The model under review builds one solid part; all positions refer to its coordinate system, in mm. A direction names the side the tool comes from. Coordinates: 2 decimals unless noted, no trailing zeros. Loops run counter-clockwise (first coordinate to the right, second up) from the corner with the lowest first, then second, coordinate; pieces in that order, holes last. Notation, with made-up numbers: (59.25, -37.5) - (74.25, -37.5) arc R15 ccw to (74.25, -12.5) - close; hole circle Ø8 at (22, -27). An arc over 180 degrees is marked (long way). Use a Markdown table: item, result. Add a question column.
1) To check wall thickness, follow L1, parallel to X at y = 2.7, z = -36.5; L2, parallel to X at y = 5.25, z = 0; L3, parallel to Z at x = -25, y = 1.35. State the ranges of each line that lie inside material, in increasing order. Write a range as [from, to].
2) The part is to be moulded in two halves that separate along Z. For faces 4 (the cylindrical face through (25.428, 1.972, 2.556)), 5 (the flat face through (0, 0, -19)), 6 (the flat face through (-18.5, 7.5, -2.6)), say which applies: pulls with the +Z half, pulls with the -Z half, needs draft (parallel to the pull), parting line crosses it, or undercut.
3) Clearance check with flat-ended pins moving along their axes: pin 1 (2.5 mm diameter, centred on y = 8, z = 0, fed in from -X); pin 2 (6.5 mm diameter, centred on x = -25, z = -36.5, fed in from +Y); pin 3 (1.5 mm diameter, centred on y = 8, z = 0.5, fed in from +X). State where each tip first meets the part, or that it passes through.
4) Add section D-D, the plane z = 11. Give the boundary of the cut face in (x, y), and give its area (3 significant figures).
5) Add section A-A, the plane y = 7.75. Give the boundary of the cut face in (x, z), and give its area (3 significant figures).
6) For faces 1 (the flat face through (21.5, 7.5, 2.6)), 2 (the flat face through (21.5, 7.5, -2.6)), 3 (the flat face through (23, 8, 0)), list the 3-axis set-ups (+Z, -Z, +X, -X, +Y, -Y) from which the entire face can be reached by the end or side of a thin tool; tool diameter is ignored.
7) Add section B-B, the plane z = 0. Give the boundary of the cut face in (x, y), and give its area (3 significant figures).
8) Add section C-C, the plane x = 1. Give the boundary of the cut face in (y, z), and give its area (3 significant figures).
```python
from build123d import *

# Parameters (mm, degrees)
SKETCH1_R           = 14
SKETCH1_R_2         = 2.5
BOSS_EXTRUDE1_DEPTH = 4
FILLET1_R           = 3
SKETCH2_R           = 1.5
CUT_EXTRUDE1_DEPTH  = 10
BOSS_EXTRUDE2_START = 5
SKETCH3_R           = 1.5
BOSS_EXTRUDE2_DEPTH = 5
FILLET2_R           = 2
BOSS_EXTRUDE3_DEPTH = 4


with BuildPart() as part:
    # Sketch1 → Boss-Extrude1 (new body)
    with BuildSketch(Plane(origin=(0, 0, 0), x_dir=(1, 0, 0), z_dir=(0, 1, 0))):
        with BuildLine():
            Line((8.126919667, 17.174200905), (19.588621549, 33.908285652))
            ThreePointArc((19.588621549, 33.908285652), (28.390534034, 41.45017969), (24.538801239, 30.517751618))
            Line((24.538801239, 30.517751618), (13.077099357, 13.783666871))
            ThreePointArc((13.077099357, 13.783666871), (16.116177061, 10.06324187), (18.125, 5.699506558))
            ThreePointArc((18.125, 5.699506558), (26, 0), (18.125, -5.699506558))
            ThreePointArc((18.125, -5.699506558), (11.240760103, -15.318136711), (0, -19))
            ThreePointArc((0, -19), (-11.240760103, -15.318136711), (-18.125, -5.699506558))
            ThreePointArc((-18.125, -5.699506558), (-26, 0), (-18.125, 5.699506558))
            ThreePointArc((-18.125, 5.699506558), (-16.116177061, 10.06324187), (-13.077099357, 13.783666871))
            Line((-13.077099357, 13.783666871), (-24.538801239, 30.517751618))
            ThreePointArc((-24.538801239, 30.517751618), (-28.390534034, 41.45017969), (-19.588621549, 33.908285652))
            Line((-19.588621549, 33.908285652), (-8.126919667, 17.174200905))
            ThreePointArc((-8.126919667, 17.174200905), (0, 19), (8.126919667, 17.174200905))
        make_face()
        with Locations(Location((0, 0, 0), (0, 0, 270))):
            Circle(SKETCH1_R, mode=Mode.SUBTRACT)
        with Locations(Location((25, 36.5, 0), (0, 0, 270))):
            Circle(SKETCH1_R_2, mode=Mode.SUBTRACT)
        with Locations(Location((-25, 36.5, 0), (0, 0, 90))):
            Circle(SKETCH1_R_2, mode=Mode.SUBTRACT)
    extrude(amount=BOSS_EXTRUDE1_DEPTH)

    # Fillet1
    fillet1_edges = [part.edges().sort_by_distance(p)[0] for p in [
        (8.126919667, 2, -17.174200905),
        (19.588621549, 2, -33.908285652),
        (24.538801239, 2, -30.517751618),
        (13.077099357, 2, -13.783666871),
        (18.125, 2, 5.699506558),
        (-18.125, 2, 5.699506558),
        (-18.125, 2, -5.699506558),
        (-13.077099357, 2, -13.783666871),
        (-24.538801239, 2, -30.517751618),
        (-19.588621549, 2, -33.908285652),
        (-8.126919667, 2, -17.174200905),
    ]]
    fillet(fillet1_edges, radius=FILLET1_R)

    # Sketch2 → Cut-Extrude1 (cut)
    with BuildSketch(Plane(origin=(0, 4, 0), x_dir=(1, 0, 0), z_dir=(0, 1, 0))):
        with Locations(Location((20, 0, 0), (0, 0, 270))):
            Circle(SKETCH2_R)
        with Locations(Location((-20, 0, 0), (0, 0, 90))):
            Circle(SKETCH2_R)
    extrude(amount=-CUT_EXTRUDE1_DEPTH, mode=Mode.SUBTRACT)

    # Sketch3 → Boss-Extrude2 (add)
    # profile 1 of 2: a face of its own
    with BuildSketch(Plane(origin=(0, 4, 0), x_dir=(1, 0, 0), z_dir=(0, 1, 0)).offset(BOSS_EXTRUDE2_START)):
        Polygon((-20, 3.464101615), (-23, 1.732050808), (-23, -1.732050808), (-20, -3.464101615), (-17, -1.732050808), (-17, 1.732050808), align=None)
        with Locations(Location((-20, 0, 0), (0, 0, 270))):
            Circle(SKETCH3_R, mode=Mode.SUBTRACT)
    # profile 2 of 2: a face of its own
    with BuildSketch(Plane(origin=(0, 4, 0), x_dir=(1, 0, 0), z_dir=(0, 1, 0)).offset(BOSS_EXTRUDE2_START)):
        Polygon((20, 3.464101615), (17, 1.732050808), (17, -1.732050808), (20, -3.464101615), (23, -1.732050808), (23, 1.732050808), align=None)
        with Locations(Location((20, 0, 0), (0, 0, 270))):
            Circle(SKETCH3_R, mode=Mode.SUBTRACT)
    extrude(amount=-BOSS_EXTRUDE2_DEPTH)

    # Fillet2
    fillet2_edges = [part.edges().sort_by_distance(p)[0] for p in [
        (-18.5, 4, -2.598076211),
        (-21.5, 4, -2.598076211),
        (-23, 4, 0),
        (-21.5, 4, 2.598076211),
        (-18.5, 4, 2.598076211),
        (-17, 4, 0),
        (21.5, 4, -2.598076211),
        (18.5, 4, -2.598076211),
        (17, 4, 0),
        (18.5, 4, 2.598076211),
        (21.5, 4, 2.598076211),
        (23, 4, 0),
    ]]
    fillet(fillet2_edges, radius=FILLET2_R)

    # Sketch4 → Boss-Extrude3 (add)
    with BuildSketch(Plane(origin=(0, 4, 0), x_dir=(1, 0, 0), z_dir=(0, 1, 0))):
        with BuildLine():
            ThreePointArc((24.772139191, 3.636851323), (20.864321919, 18.474065491), (28.618293037, 31.7137744))
            ThreePointArc((28.618293037, 31.7137744), (21.354403975, 32.800609697), (20.161290323, 40.047800538))
            ThreePointArc((20.161290323, 40.047800538), (0, 29.83030278), (-20.161290323, 40.047800538))
            ThreePointArc((-20.161290323, 40.047800538), (-21.354403975, 32.800609697), (-28.618293037, 31.7137744))
            ThreePointArc((-28.618293037, 31.7137744), (-20.864321919, 18.474065491), (-24.772139191, 3.636851323))
            ThreePointArc((-24.772139191, 3.636851323), (-19.807252921, 3.994836175), (-15.415783274, 6.338603052))
            ThreePointArc((-15.415783274, 6.338603052), (-9.04861994, 13.254364925), (0, 15.802110673))
            ThreePointArc((0, 15.802110673), (9.04861994, 13.254364925), (15.415783274, 6.338603052))
            ThreePointArc((15.415783274, 6.338603052), (19.807252921, 3.994836175), (24.772139191, 3.636851323))
        make_face()
    extrude(amount=-BOSS_EXTRUDE3_DEPTH)


solid = part.part
```
From the geometry:
| question | item | result |
|---|---|---|
| 1 | L1 | x = [-31, -27.5], [-22.5, -17], [17, 22.5], [27.5, 31] |
| 1 | L2 | x = [-23.15, -21.5], [-18.5, -16.85], [16.85, 18.5], [21.5, 23.15] |
| 1 | L3 | z = [-42.5, -39], [-34, -28.18], [-3.32, 3.32] |
| 2 | face 4 | undercut |
| 2 | face 5 | needs draft |
| 2 | face 6 | pulls with the -Z half |
| 3 | pin 1 | stops at x = -23 |
| 3 | pin 2 | stops at y = 4 |
| 3 | pin 3 | stops at x = 23 |
| 4 | outline | (-15.49, 0) - (-8.66, 0) - (-8.66, 4) - (-15.49, 4) - close; (8.66, 0) - (15.49, 0) - (15.49, 4) - (8.66, 4) - close |
| 4 | area | 54.7 mm^2 |
| 5 | outline | (-23, -1.73) - (-20, -3.46) - (-17, -1.73) - (-17, 1.73) - (-20, 3.46) - (-23, 1.73) - close; (17, -1.73) - (20, -3.46) - (23, -1.73) - (23, 1.73) - (20, 3.46) - (17, 1.73) - close; hole circle Ø3 at (-20, 0); hole circle Ø3 at (20, 0) |
| 5 | area | 48.2 mm^2 |
| 6 | face 1 | +Z, +X, +Y |
| 6 | face 2 | -Z, +X, +Y |
| 6 | face 3 | +Z, -Z, +X, +Y |
| 7 | outline | (-26, 0) - (-21.5, 0) - (-21.5, 9) - (-23, 9) - (-23, 6) arc R2 cw to (-25, 4) - (-26, 4) - close; (-18.5, 0) - (-14, 0) - (-14, 4) - (-15, 4) arc R2 cw to (-17, 6) - (-17, 9) - (-18.5, 9) - close; (14, 0) - (18.5, 0) - (18.5, 9) - (17, 9) - (17, 6) arc R2 cw to (15, 4) - (14, 4) - close; (21.5, 0) - (26, 0) - (26, 4) - (25, 4) arc R2 cw to (23, 6) - (23, 9) - (21.5, 9) - close |
| 7 | area | 105 mm^2 |
| 8 | outline | (0, -29.85) - (4, -29.85) - (4, -13.96) - (0, -13.96) - close; (0, 13.96) - (4, 13.96) - (4, 18.97) - (0, 18.97) - close |
| 8 | area | 83.6 mm^2 |
